from build123d import *

# Parameters (mm, degrees)
F0_R     = 25
F1_DEPTH = 3
F2_R     = 1.75
F3_DEPTH = 1
F4_R     = 1.75
F5_DEPTH = 1
F7_DEPTH = 25


with BuildPart() as f1:
    # F0 (on Top) → F1 (new body)
    with BuildSketch(Plane.XY):
        Circle(F0_R)
    extrude(amount=F1_DEPTH)

    # F2 (on face) → F3 (cut)
    with BuildSketch(Plane.XY.offset(3)):
        with BuildLine():
            ThreePointArc((0, -25), (17.67767, -17.67767), (25, 0))
            ThreePointArc((25, 0), (17.67767, 17.67767), (0, 25))
            ThreePointArc((0, 25), (-9.429286, 12.5), (0, 0))
            ThreePointArc((0, 0), (9.429286, -12.5), (0, -25))
        make_face()
        with Locations((3.570714, 12.5)):
            Circle(F2_R, mode=Mode.SUBTRACT)
        with Locations((-3.570714, -12.5)):
            Circle(F2_R)
    extrude(amount=-F3_DEPTH, mode=Mode.SUBTRACT)

    # F4 (on face) → F5 (cut)
    with BuildSketch(Plane(origin=(0, 0, 0), x_dir=(1, 0, 0), z_dir=(0, 0, -1))):
        with BuildLine():
            ThreePointArc((0, 0), (9.429286, 12.5), (0, 25))
            ThreePointArc((0, 25), (-25, 0), (0, -25))
            ThreePointArc((0, -25), (-9.429286, -12.5), (0, 0))
        make_face()
        with Locations((-3.570714, 12.5)):
            Circle(F4_R, mode=Mode.SUBTRACT)
        with Locations((3.570714, -12.5)):
            Circle(F4_R)
    extrude(amount=-F5_DEPTH, mode=Mode.SUBTRACT)

    # F6 (on face) → F7 (cut)
    with BuildSketch(Plane.XY.offset(3)):
        with BuildLine():
            ThreePointArc((0, 0), (-0.478127, 0.146584), (-0.950263, 0.311449))
            ThreePointArc((-0.950263, 0.311449), (-0.311449, -0.950263), (0.950263, -0.311449))
            ThreePointArc((0.950263, -0.311449), (0.478127, -0.146584), (0, 0))
        make_face()
        with BuildLine():
            ThreePointArc((0.950263, -0.311449), (0.987487, -0.157698), (1, 0))
            ThreePointArc((1, 0), (0.157698, 0.987487), (-0.950263, 0.311449))
            ThreePointArc((-0.950263, 0.311449), (-0.478127, 0.146584), (0, 0))
            ThreePointArc((0, 0), (0.478127, -0.146584), (0.950263, -0.311449))
        make_face()
    extrude(amount=-F7_DEPTH, mode=Mode.SUBTRACT)


solid = f1.part
The listing builds one solid part. Answer for the finished solid, in the listing's coordinates (mm). A direction names the side the tool comes from. Round coordinates to 2 decimals unless told otherwise and drop trailing zeros. Order: outer loops, then holes, each group sorted by start corner. A loop starts at its lowest first (then second) coordinate and runs counter-clockwise, first axis right, second up. Notation, with made-up numbers: M 30,66.25 L 49,66.25 A18 ccw 49,101.25 Z; hole C 3.25,19 d9. An arc over 180 degrees is marked long. Answer in a Markdown table with one row per item. Add a question column.
1) Determine the mould class of faces 4 (the face through (23.09, -9.58, 1.48)), 5 (the face through (3.343, 10.765, 0.493)), 6 (the face through (-8, -5, 3)) for opening direction Y: pulls with the +Y half, pulls with the -Y half, needs draft (parallel to the pull), parting line crosses it, or undercut.
2) The part is cut by section A-A on x = -20. Determine the outline of the cut face in (y, z).
3) Which of the six approach directions +Z, -Z, +X, -X, +Y, -Y give full straight-line access (tool end or side, diameter ignored) to faces 1 (the face through (-3.799, -14.235, 0.493)), 2 (the face through (-3.799, -10.765, 2.507)), 3 (the face through (9.426, -12.772, 2.507))?
4) The part is cut by section D-D on x = 8.5. Determine the outline of the cut face in (y, z), plus the area to 3 significant figures.
5) The part is cut by section B-B on y = 12.5. Determine the outline of the cut face in (x, z).
6) Consider line 1 along Z through (x, y) = (-16, -16); line 2 along Z through (x, y) = (14, -16); line 3 along Y through (x, z) = (1.5, 0.75). Determine where each line is inside the solid, lowest interval first. Write a range as from..to.
7) Flat-ended cylindrical pins translate along their axes: pin 1 Ø10.5 at (x, y) = (-15, 4.5) entering from -Z; pin 2 Ø1.5 at (x, z) = (-2.5, 2.5) entering from +Y; pin 3 Ø6 at (x, y) = (19.5, 4) entering from +Z. Find the tip coordinate at first contact, or state that the pin passes through.
8) The part is cut by section C-C on z = 1.45. Determine the outline of the cut face in (x, y), plus the area to 3 significant figures.
Findings below:
| question | item | result |
|---|---|---|
| 1 | face 4 | parting line crosses it |
| 1 | face 5 | undercut |
| 1 | face 6 | needs draft |
| 2 | outline | M -15,1 L 15,1 L 15,3 L -15,3 Z |
| 3 | face 1 | -Z |
| 3 | face 2 | +Z |
| 3 | face 3 | +Z, +X |
| 4 | outline | M -23.51,0 L -17.33,0 L -17.33,1 L -7.67,1 L -7.67,0 L 23.51,0 L 23.51,2 L -7.67,2 L -7.67,3 L -17.33,3 L -17.33,2 L -23.51,2 Z |
| 4 | area | 94.0 mm² |
| 5 | outline | M -21.65,1 L -9.43,1 L -9.43,0 L 1.82,0 L 1.82,1 L 5.32,1 L 5.32,0 L 21.65,0 L 21.65,2 L 5.32,2 L 5.32,3 L 1.82,3 L 1.82,2 L -9.43,2 L -9.43,3 L -21.65,3 Z |
| 6 | line 1 | z = 1..3 |
| 6 | line 2 | z = 0..2 |
| 6 | line 3 | y = -24.95..-24.47, -0.53..24.95 |
| 7 | pin 1 | stops at z = 1 |
| 7 | pin 2 | stops at y = 24.94 |
| 7 | pin 3 | stops at z = 2 |
| 8 | outline | C 0,0 d50; hole M 0.95,-0.31 A1 ccw 1,0 A1 ccw long Z |
| 8 | area | 1,960 mm² |
